from build123d import *

# Parameters (mm, degrees)
SKETCH1_W           = 202.5
SKETCH1_H           = 20
SKETCH1_R           = 3
BOSS_EXTRUDE1_DEPTH = 50
SKETCH2_W           = 80
SKETCH2_H           = 31
SKETCH2_W_2         = 147.5
SKETCH2_H_2         = 10
CUT_EXTRUDE1_DEPTH  = 25
CHAMFER1_SIZE       = 10
FILLET1_R           = 10
FILLET2_START       = -10
FILLET2_DEPTH       = 20


with BuildPart() as part:
    # Sketch1 → Boss-Extrude1 (new body)
    with BuildSketch(Plane(origin=(0, 0, 0), x_dir=(1, 0, 0), z_dir=(0, 1, 0))):
        Rectangle(SKETCH1_W, SKETCH1_H)
        with Locations(Location((-91.25, 0, 0), (0, 0, 270))):
            Circle(SKETCH1_R, mode=Mode.SUBTRACT)
        with Locations(Location((88.75, 0, 0), (0, 0, 270))):
            Circle(SKETCH1_R, mode=Mode.SUBTRACT)
    extrude(amount=BOSS_EXTRUDE1_DEPTH)

    # Sketch2 → Cut-Extrude1 (cut)
    with BuildSketch(Plane.XY.offset(10)):
        with Locations((101.25, 25)):
            Rectangle(SKETCH2_W, SKETCH2_H)
        with Locations((-27.5, 45)):
            Rectangle(SKETCH2_W_2, SKETCH2_H_2)
        with Locations((-27.5, 5)):
            Rectangle(SKETCH2_W_2, SKETCH2_H_2)
    extrude(amount=-CUT_EXTRUDE1_DEPTH, mode=Mode.SUBTRACT)

    # Chamfer1
    chamfer1_edges = [part.edges().sort_by_distance(p)[0] for p in [
        (46.25, 0, 0),
        (46.25, 50, 0),
    ]]
    chamfer(chamfer1_edges, length=CHAMFER1_SIZE - 0.0001)  # a hair under: the kernel refuses the full size

    # Fillet1
    fillet1_edges = [part.edges().sort_by_distance(p)[0] for p in [
        (61.25, 9.5, 0),
        (61.25, 40.5, 0),
    ]]
    fillet(fillet1_edges, radius=FILLET1_R)

    # Fillet2: read off the stored shape, not the designer's step
    # Fillet2 outline → Fillet2 (add)
    with BuildSketch(Plane.XY.offset(FILLET2_START)):
        with BuildLine():
            ThreePointArc((49.178932188, 42.928932188), (45.9346987, 40.761204675), (42.107864376, 40))
            Line((42.107864376, 40), (46.25, 40))
            Line((46.25, 40), (49.178932188, 42.928932188))
        make_face()
        with BuildLine():
            Line((46.25, 10), (42.107864376, 10))
            ThreePointArc((42.107864376, 10), (45.9346987, 9.238795325), (49.178932188, 7.071067812))
            Line((49.178932188, 7.071067812), (46.25, 10))
        make_face()
    extrude(amount=FILLET2_DEPTH)


solid = part.part
Could you check a few things on this model? Use its own coordinates, in mm. A direction names the side the tool comes from. Give positions to 0.01 mm unless a question says otherwise; leave off trailing zeros. Order: outer loops, then holes, each group sorted by start corner. A loop starts at its lowest first (then second) coordinate and runs counter-clockwise, first axis right, second up.
1. Suppose I cut it at C-C (y = 22.5). List the corners of the cut face in (x, z) for me.
2. Suppose I cut it at A-A (z = 0). List the corners of the cut face in (x, y) for me, plus the area to 3 significant figures.
3. Suppose I cut it at D-D (z = 8.25). List the corners of the cut face in (x, y) for me, plus the area to 3 significant figures.
4. Will these pins go through, and if not, where does the flat tip stop? P1, Ø3.5, axis at y = 23.5, z = 3, coming from the +X side; P2, Ø3.5, axis at x = 88.75, z = 0, coming from the -Y side; P3, Ø6, axis at y = 32.5, z = 6, coming from the +X side; P4, Ø6, axis at x = 22, z = 0, coming from the -Y side.
5. Suppose I cut it at B-B (x = 75). List the corners of the cut face in (y, z) for me.
6. I need wall thicknesses on L1, parallel to Y at x = 93, z = -3.5; L2, parallel to Z at x = 88.75, y = 46.75; L3, parallel to Y at x = -75.5, z = -1. Which ranges of each line are inside material? Lowest first, please.
7. For faces 4 (the flat face through (-31, 40, 0)), 5 (the cylindrical face through (64.26, 12.35, -0.14)), 6 (the flat face through (-101.25, 25, 0)), which set-ups out of +Z, -Z, +X, -X, +Y, -Y let a thin tool reach every point of the face, with its end or its side?
8. We'd pull the mould along X, two halves only. Please class faces 1 (the cylindrical face through (-94.18, 24.79, -0.65)), 2 (the cylindrical face through (45.968, 40.775, -0.14)), 3 (the flat face through (-31, 10, 0)): pulls with the +X half, pulls with the -X half, needs draft (parallel to the pull), parting line crosses it, or undercut.
Solved:
1. outline: (-101.25, -10) - (61.25, -10) - (61.25, 10) - (-101.25, 10) - close; hole circle Ø6 at (-91.25, 0)
2. outline: (-101.25, 10) - (-94.25, 10) - (-94.25, 40) - (-101.25, 40) - close; (-88.25, 10) - (42.11, 10) arc R10 cw to (49.15, 7.1) - (56.25, 0) - (85.75, 0) - (85.75, 9.5) - (71.25, 9.5) arc R10 cw to (61.25, 19.5) - (61.25, 30.5) arc R10 cw to (71.25, 40.5) - (85.75, 40.5) - (85.75, 50) - (56.25, 50) - (49.15, 42.9) arc R10 cw to (42.11, 40) - (-88.25, 40) - close; (91.75, 0) - (101.25, 0) - (101.25, 9.5) - (91.75, 9.5) - close; (91.75, 40.5) - (101.25, 40.5) - (101.25, 50) - (91.75, 50) - close
2. area: 5,590 mm2
3. outline: (-101.25, 10) - (42.11, 10) arc R10 cw to (49.15, 7.1) - (56.25, 0) - (101.25, 0) - (101.25, 9.5) - (71.25, 9.5) arc R10 cw to (61.25, 19.5) - (61.25, 30.5) arc R10 cw to (71.25, 40.5) - (101.25, 40.5) - (101.25, 50) - (56.25, 50) - (49.15, 42.9) arc R10 cw to (42.11, 40) - (-101.25, 40) - close
3. area: 5,880 mm2
4. P1: stops at x = 61.25
4. P2: passes through
4. P3: stops at x = 62.59
4. P4: stops at y = 10
5. outline: (0, -10) - (9.5, -10) - (9.5, 10) - (0, 10) - close; (40.5, -10) - (50, -10) - (50, 10) - (40.5, 10) - close
6. L1: y = 0 to 9.5, 40.5 to 50
6. L2: z = -10 to -3, 3 to 10
6. L3: y = 10 to 40
7. face 4: +Z, -Z, -X, +Y
7. face 5: +Z, -Z, +X
7. face 6: +Z, -Z, -X, +Y, -Y
8. face 1: undercut
8. face 2: pulls with the -X half
8. face 3: needs draft
